Source: CAD feature listing. Evaluate the final solid. Frame: model axes, mm. A direction names the side the tool comes from. Give positions to 0.01 mm unless a question says otherwise; leave off trailing zeros. Order: outer loops, then holes, each group sorted by start corner. A loop starts at its lowest first (then second) coordinate and runs counter-clockwise, first axis right, second up.
from build123d import *

# Parameters (mm, degrees)
F1_DEPTH = 40


with BuildPart() as f1:
    # F0 (on Front) → F1 (new body)
    with BuildSketch(Plane.XZ):
        Polygon((0, -44.541744), (0, 0), (-400, 0), (-400, 1000), (-440, 1000), (-440, 0), (-440, -592.545841), (-400, -592.545841), (-400, -44.541744), align=None)
        Polygon((400, 0), (0, 0), (0, -44.541744), (400, -44.541744), (400, -592.545841), (440, -592.545841), (440, 0), (440, 1000), (400, 1000), align=None)
    extrude(amount=F1_DEPTH)


solid = f1.part
1) First-contact query: pin 1 Ø12 at (x, y) = (47, -11.5) entering from +Z; pin 2 Ø10 at (x, y) = (-24, -27) entering from -Z. Flat tips, straight axial feed; report the tip coordinate or a pass-through.
Checks:
pin 1: stops at z = 0
pin 2: stops at z = -44.54
2) Pull-direction query (X, two-part tool) for faces 1 (the face through (-440, -20, 215)), 2 (the face through (-420, -20, -592.546)), 3 (the face through (-400, -20, 493)); classes: +X half, -X half, draft (parallel to the pull), parting line (faces both ways), or undercut.
Checks:
face 1: -X half
face 2: draft
face 3: undercut
3) Ray query, L1, parallel to X at y = -24, z = 884; L2, parallel to Z at x = -1, y = -12. Return the intervals inside material, ascending.
Checks:
L1: x = -440 to -400, 400 to 440
L2: z = -44.54 to 0
4) Section query C-C on x = -152. Output: boundary loops of the cut face in (y, z).
Checks:
outline: (-40, -44.54) - (0, -44.54) - (0, 0) - (-40, 0) - close
5) Section query B-B on y = -34. Output: boundary loops of the cut face in (x, z), and give its area (3 significant figures).
Checks:
outline: (-440, -592.55) - (-400, -592.55) - (-400, -44.54) - (400, -44.54) - (400, -592.55) - (440, -592.55) - (440, 1000) - (400, 1000) - (400, 0) - (-400, 0) - (-400, 1000) - (-440, 1000) - close
area: 163,000 mm2
6) Section query A-A on z = -287. Output: boundary loops of the cut face in (x, y).
Checks:
outline: (-440, -40) - (-400, -40) - (-400, 0) - (-440, 0) - close; (400, -40) - (440, -40) - (440, 0) - (400, 0) - close
7) Reachability of faces 4 (the face through (6, -20, 0)), 5 (the face through (400, -20, -315)), 6 (the face through (420, -20, 1000)) from +Z, -Z, +X, -X, +Y, -Y: full face, straight path, thin tool, end or side. Return the list, or none.
Checks:
face 4: +Z, +Y, -Y
face 5: -Z, +Y, -Y
face 6: +Z, +X, -X, +Y, -Y
